Autodesk Inventor part; units mm, degrees
ref_plane "YZ Plane" through (0, 0, 0) normal (1, 0, 0) x (0, 1, 0)
ref_plane "XZ Plane" through (0, 0, 0) normal (0, 1, 0) x (-1, 0, 0)
ref_plane "XY Plane" through (0, 0, 0) normal (0, 0, 1) x (1, 0, 0)
sketch "Sketch1" plane through (0, 0, 0) normal (0, 1, 0) x (-1, 0, 0)
  line L0 (0, 0) -> (9.5, 0)
  line L1 (9.5, 0) -> (9.5, -64)
  line L2 (9.5, -64) -> (0, -64)
  line L3 (0, -64) -> (0, 0)
  circle A0 centre (3.7, -11.5) radius 2.25
  circle A1 centre (3.7, -59.5) radius 2.25
  line L4 (3.7, -11.5) -> (3.7, -59.5) construction
  dimension "d1" = 9.5
  dimension "d2" = 64
  dimension "d3" = 4.5
  dimension "d4" = 48
  dimension "d6" = 3.7
  dimension "d17" = 4.5
extrude "Extrusion1" add sketch "Sketch1" along normal blind 12
sketch "Sketch2" plane through (-9.5, 0, 0) normal (0, 0, 1) x (1, 0, 0)
  line L0 (9.5, 12) -> (0, 12)
  line L1 (3, 12) -> (8.4, 12)
  line L2 (8.4, 12) -> (8.4, 10.8)
  line L3 (8.4, 10.8) -> (3, 10.8)
  line L4 (3, 10.8) -> (3, 12)
  line L5 (9.5, 0) -> (9.5, 12)
  line L6 (3.55, 0) -> (8.05, 0)
  line L7 (3.55, 12) -> (8.05, 12)
  line L8 (9.5, 0) -> (9.5, 12)
  line L9 (9.5, 0) -> (9.5, 12)
  line L10 (3.55, 12) -> (8.05, 12)
  line L11 (3.55, 12) -> (3.55, 0)
  line L12 (3.55, 12) -> (8.05, 12)
  line L13 (3.55, 0) -> (8.05, 0)
  line L14 (3.55, 12) -> (8.05, 12)
  line L15 (3.55, 0) -> (8.05, 0)
  line L16 (3.55, 12) -> (8.05, 12)
  line L17 (3.55, 0) -> (8.05, 0)
  dimension "d9" = 1.1
  dimension "d10" = 5.4
  dimension "d11" = 1.2
  dimension "d76" = 12
extrude "Extrusion2" cut sketch "Sketch2" against normal up to next
sketch "Sketch3" plane through (0, 0, 0) normal (0, -1, 0) x (1, 0, 0)
  circle A0 centre (-3.7, -11.5) radius 2.25
  circle A1 centre (-3.7, -11.5) radius 3.75
  circle A2 centre (-3.7, -59.5) radius 2.25
  circle A3 centre (-3.7, -59.5) radius 3.75
  point P0 (0, 0)
  dimension "d14" = 7.5
extrude "Extrusion3" cut sketch "Sketch3" against normal blind 3
fillet "Fillet1" radius 1 4 edges at (0, 1.5, -58.8897) (0, 1.5, -60.1103) (0, 1.5, -10.8897) (0, 1.5, -12.1103)
fillet "Fillet2" radius 4 2 edges at (-9.5, 6, -64) (-9.5, 6, 0)
sketch "Sketch15" plane through (0, 0, 0) normal (0, -1, 0) x (1, 0, 0)
  line L0 (0, 0) -> (0, -7.592)
  line L1 (-9.5, -32) -> (-9.5, -21)
  line L2 (-9.5, -21) -> (0, -21)
  line L3 (0, -21) -> (0, -43)
  line L4 (0, -43) -> (-9.5, -43)
  line L5 (-9.5, -43) -> (-9.5, -32)
  dimension "d79" = 11
  dimension "d80" = 22
extrude "Extrusion15" add sketch "Sketch15" along normal blind 15
sketch "Sketch16" plane through (0, -15, 0) normal (0, -1, 0) x (1, 0, 0)
  line L0 (-9.5, -43) -> (0, -43)
  line L1 (0, -43) -> (-60, -43)
  line L2 (-60, -43) -> (-60, -33)
  line L3 (-60, -33) -> (0, -33)
  line L4 (0, -33) -> (0, -43)
  point P0 (0, 0)
  dimension "d83" = 60
  dimension "d84" = 10
  dimension "d85" = 60
extrude "Extrusion16" add sketch "Sketch16" along normal blind 10
properties part number "Back_base"
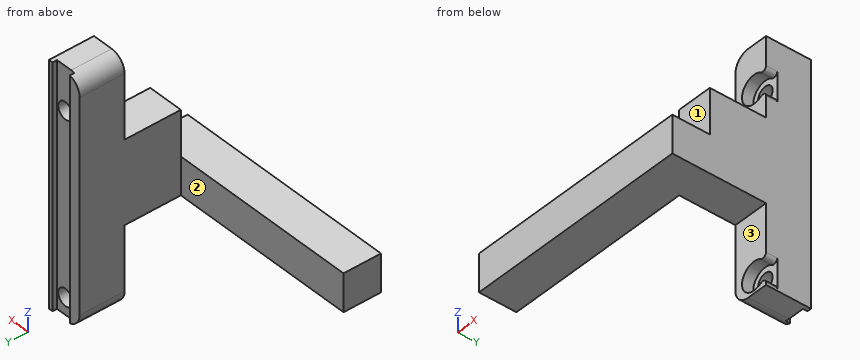
Geometry: final body of the model. Coordinates: model frame, mm. Face numbers are marked on the shaded views. A direction names the side the tool comes from. Give positions to 0.01 mm unless a question says otherwise; leave off trailing zeros. Order: outer loops, then holes, each group sorted by start corner. A loop starts at its lowest first (then second) coordinate and runs counter-clockwise, first axis right, second up. Notation, with made-up numbers: (-28, 1) -> (18, 1) arc R12 ccw to (18, 17) -> close; hole circle Ø11 at (10, 1.5). An arc over 180 degrees is marked (long way). Put each result on its own line as item: value.
Q1. Section C-C, the plane x = -3.7. Return loops of the section in (y, z), then the cut area to 3 significant figures.
Here are the results:
outline: (-25, -43) -> (0, -43) -> (0, -55.75) -> (3, -55.75) -> (3, -57.25) -> (10.8, -57.25) -> (10.8, -13.75) -> (3, -13.75) -> (3, -15.25) -> (0, -15.25) -> (0, -21) -> (-15, -21) -> (-15, -33) -> (-25, -33) -> close; (0, -64) -> (10.8, -64) -> (10.8, -61.75) -> (3, -61.75) -> (3, -63.25) -> (0, -63.25) -> close; (0, -7.75) -> (3, -7.75) -> (3, -9.25) -> (10.8, -9.25) -> (10.8, 0) -> (0, 0) -> close
area: 1,010 mm^2
Q2. Section B-B, the plane z = -11.5. Return loops of the section in (x, y).
Here are the results:
outline: (-9.5, 0) -> (-7.45, 0) -> (-7.45, 3) -> (-5.95, 3) -> (-5.95, 10.8) -> (-6.5, 10.8) -> (-6.5, 12) -> (-9.5, 12) -> close; (-1.45, 3) -> (0, 3) -> (0, 12) -> (-1.1, 12) -> (-1.1, 10.8) -> (-1.45, 10.8) -> close
Q3. Reachability of the marked faces 1, 2 and 3 from +Z, -Z, +X, -X, +Y, -Y: full face, straight path, thin tool, end or side. Return the list, or none.
Here are the results:
face 1: +Z, +X, -X, -Y
face 2: +Z, -Z, -X, +Y
face 3: -Z, +X, -X, -Y
Q4. Section A-A, the plane y = 7. Return loops of the section in (x, z).
Here are the results:
outline: (-9.5, -60) arc R4 ccw to (-5.5, -64) -> (0, -64) -> (0, 0) -> (-5.5, 0) arc R4 ccw to (-9.5, -4) -> close; hole circle Ø4.5 at (-3.7, -59.5); hole circle Ø4.5 at (-3.7, -11.5)
Q5. Material intervals for L1, parallel to Z at x = -3.7, y = 7.25; L2, parallel to Z at x = -3.7, y = 2.25; L3, parallel to X at y = 7, z = -11.5, sorted ascending.
Here are the results:
L1: z = -64 to -61.75, -57.25 to -13.75, -9.25 to 0
L2: z = -64 to -63.25, -55.75 to -15.25, -7.75 to 0
L3: x = -9.5 to -5.95, -1.45 to 0
Q6. Pin query (flat end, axial travel): pin 1 (1 mm diameter, centred on x = -53.5, z = -31.5, fed in from +Y); pin 2 (5 mm diameter, centred on x = -3.5, z = -25.5, fed in from -Y); pin 3 (7 mm diameter, centred on x = -3.7, z = -11.5, fed in from -Y); pin 4 (7.5 mm diameter, centred on x = -4.5, z = -48.5, fed in from -Y). Return the tip coordinate at first contact, or that it passes through.
Here are the results:
pin 1: passes through
pin 2: stops at y = -15
pin 3: stops at y = 3
pin 4: stops at y = 0
Q7. Section D-D, the plane z = -38. Return loops of the section in (x, y).
Here are the results:
outline: (-60, -25) -> (0, -25) -> (0, 12) -> (-1.1, 12) -> (-1.1, 10.8) -> (-6.5, 10.8) -> (-6.5, 12) -> (-9.5, 12) -> (-9.5, -15) -> (-60, -15) -> close
